CAD build for the part. Positions are in the model's coordinates, mm. A direction names the side the tool comes from. Round coordinates to 2 decimals unless told otherwise and drop trailing zeros. Write each loop counter-clockwise with the first axis right and the second up, starting at its lowest first coordinate (ties: lowest second). Pieces come first, ordered by that corner, then holes. Notation, with made-up numbers: (81.25, 71.25) -> (101.25, 71.25) arc R26 ccw to (101.25, 91.25) -> close; hole circle Ø7 at (14.25, 75.25). An arc over 180 degrees is marked (long way). Put each result on its own line as item: value. Start each with the question number.
1. Saw through at D-D on z = -29. List the corners of the cut face in (x, y) (3 decimals), and give its area (3 significant figures).
2. Pull direction Y, two halves, no side cores. Call faces 1 (the cylindrical face through (-2.21, 39.84, 41.27)), 2 (the flat face through (19.685, 55, 1)), 3 (the flat face through (43, 7.79, -62)): pulls with the +Y half, pulls with the -Y half, needs draft (parallel to the pull), parting line crosses it, or undercut.
3. Flat gauge pins, fed straight in: P1, Ø2.5, axis at x = 2, z = 0.5, coming from the +Y side; P2, Ø8, axis at y = 25.5, z = -16.5, coming from the -X side; P3, Ø9, axis at x = 41.06, z = 60.58, coming from the +Y side. Where does each tip first touch, or does it go through?
4. Saw through at A-A on z = 0. List the corners of the cut face in (x, y) (3 decimals), and give its area (3 significant figures).
5. 3-axis set-ups, long thin cutter, end or side, ignore diameter. For faces 4 (the cylindrical face through (-38.927, 8.88, -63.923)), 5 (the flat face through (0, 61, 43.735)), 6 (the cylindrical face through (28.294, 13.422, -0.78)): which of +Z, -Z, +X, -X, +Y, -Y reach the whole face in a straight line?
6. Saw through at B-B on y = 61.5. List the corners of the cut face in (x, z) (3 decimals).
7. Saw through at C-C on x = 11. List the corners of the cut face in (y, z) (3 decimals).
8. Drill centre lines: line 1 (Y direction, x = 0, z = 41); line 2 (X direction, y = 77, z = -25) (3 decimals); line 3 (Z direction, x = -11.5, y = 26.5) (3 decimals). Where is each one in solid material? Low to high. Write a range as from..to.
from build123d import *

# Parameters (mm, degrees)
SKETCH1_W                                     = 49.37
SKETCH1_H                                     = 87.47
SKETCH1_W_2                                   = 39.37
SKETCH1_H_2                                   = 77.47
BOSS_EXTRUDE1_DEPTH                           = 101.6
SKETCH2_W                                     = 100.17
SKETCH2_H                                     = 138.27
BOSS_EXTRUDE2_DEPTH                           = 10
FILLET1_R                                     = 12
CBORE_FOR_6_BINDING_HEAD_MACHINE_SC_2_R       = 1.89865
CBORE_FOR_6_BINDING_HEAD_MACHINE_SCREW2_DEPTH = 10
CBORE_START                                   = 7.7902
CBORE_FOR_6_BINDING_HEAD_MACHINE_SC_3_O_R     = 3.96875
CBORE_FOR_6_BINDING_HEAD_MACHINE_SC_3_O_R_2   = 1.89865
CBORE_FOR_6_BINDING_HEAD_MACHINE_SC_3_DEPTH   = 2.2098
FILLET2_R                                     = 12
SKETCH9_R                                     = 3
CUT_EXTRUDE1_DEPTH                            = 160.908424184


# Read off the part's stored shape, not the designer's step: CBORE for #6 Binding Head Machine Screw2
with BuildPart() as part:
    # Sketch1 → Boss-Extrude1 (new body)
    with BuildSketch(Plane(origin=(0, 0, 0), x_dir=(1, 0, 0), z_dir=(0, 1, 0))):
        Rectangle(SKETCH1_W, SKETCH1_H)
        Rectangle(SKETCH1_W_2, SKETCH1_H_2, mode=Mode.SUBTRACT)
    extrude(amount=BOSS_EXTRUDE1_DEPTH)

    # Sketch2 → Boss-Extrude2 (add)
    with BuildSketch(Plane(origin=(0, 0, 0), x_dir=(1, 0, 0), z_dir=(0, 1, 0))):
        Rectangle(SKETCH2_W, SKETCH2_H)
    extrude(amount=BOSS_EXTRUDE2_DEPTH)

    # Fillet1
    fillet1_edges = [part.edges().sort_by_distance(p)[0] for p in [
        (0, 10, -43.735),
        (24.685, 10, 0),
        (0, 10, 43.735),
        (-24.685, 10, 0),
    ]]
    fillet(fillet1_edges, radius=FILLET1_R)

    # CBORE for _6 Binding Head Machine Sc 2 → CBORE for #6 Binding Head Machine Screw2 (cut)
    with BuildSketch(Plane(origin=(0, 0, 0), x_dir=(1, 0, 0), z_dir=(0, 1, 0))):
        with Locations((41.060456563, -60.576250035)):
            Circle(CBORE_FOR_6_BINDING_HEAD_MACHINE_SC_2_R)
        with Locations((-41.060456563, 60.576250035)):
            Circle(CBORE_FOR_6_BINDING_HEAD_MACHINE_SC_2_R)
        with Locations((-41.060456563, -60.576250035)):
            Circle(CBORE_FOR_6_BINDING_HEAD_MACHINE_SC_2_R)
        with Locations((41.060456563, 60.576250035)):
            Circle(CBORE_FOR_6_BINDING_HEAD_MACHINE_SC_2_R)
        Circle(CBORE_FOR_6_BINDING_HEAD_MACHINE_SC_2_R)
    extrude(amount=CBORE_FOR_6_BINDING_HEAD_MACHINE_SCREW2_DEPTH, mode=Mode.SUBTRACT)

    # CBORE for _6 Binding Head Machine Sc 3 o → CBORE for _6 Binding Head Machine Sc 3 (cut)
    # profile 1 of 5: a face of its own
    with BuildSketch(Plane(origin=(0, 0, 0), x_dir=(1, 0, 0), z_dir=(0, 1, 0)).offset(CBORE_START)):
        with Locations((41.060456563, -60.576250035)):
            Circle(CBORE_FOR_6_BINDING_HEAD_MACHINE_SC_3_O_R)
        with Locations((41.060456563, -60.576250035)):
            Circle(CBORE_FOR_6_BINDING_HEAD_MACHINE_SC_3_O_R_2, mode=Mode.SUBTRACT)
    # profile 2 of 5: a face of its own
    with BuildSketch(Plane(origin=(0, 0, 0), x_dir=(1, 0, 0), z_dir=(0, 1, 0)).offset(CBORE_START)):
        with Locations((-41.060456563, 60.576250035)):
            Circle(CBORE_FOR_6_BINDING_HEAD_MACHINE_SC_3_O_R)
        with Locations((-41.060456563, 60.576250035)):
            Circle(CBORE_FOR_6_BINDING_HEAD_MACHINE_SC_3_O_R_2, mode=Mode.SUBTRACT)
    # profile 3 of 5: a face of its own
    with BuildSketch(Plane(origin=(0, 0, 0), x_dir=(1, 0, 0), z_dir=(0, 1, 0)).offset(CBORE_START)):
        with Locations((-41.060456563, -60.576250035)):
            Circle(CBORE_FOR_6_BINDING_HEAD_MACHINE_SC_3_O_R)
        with Locations((-41.060456563, -60.576250035)):
            Circle(CBORE_FOR_6_BINDING_HEAD_MACHINE_SC_3_O_R_2, mode=Mode.SUBTRACT)
    # profile 4 of 5: a face of its own
    with BuildSketch(Plane(origin=(0, 0, 0), x_dir=(1, 0, 0), z_dir=(0, 1, 0)).offset(CBORE_START)):
        with Locations((41.060456563, 60.576250035)):
            Circle(CBORE_FOR_6_BINDING_HEAD_MACHINE_SC_3_O_R)
        with Locations((41.060456563, 60.576250035)):
            Circle(CBORE_FOR_6_BINDING_HEAD_MACHINE_SC_3_O_R_2, mode=Mode.SUBTRACT)
    # profile 5 of 5: a face of its own
    with BuildSketch(Plane(origin=(0, 0, 0), x_dir=(1, 0, 0), z_dir=(0, 1, 0)).offset(CBORE_START)):
        Circle(CBORE_FOR_6_BINDING_HEAD_MACHINE_SC_3_O_R)
        Circle(CBORE_FOR_6_BINDING_HEAD_MACHINE_SC_3_O_R_2, mode=Mode.SUBTRACT)
    extrude(amount=CBORE_FOR_6_BINDING_HEAD_MACHINE_SC_3_DEPTH, mode=Mode.SUBTRACT)

    # Fillet2
    fillet2_edges = [part.edges().sort_by_distance(p)[0] for p in [
        (50.085, 5, 69.135),
        (50.085, 5, -69.135),
        (-50.085, 5, -69.135),
        (-50.085, 5, 69.135),
    ]]
    fillet(fillet2_edges, radius=FILLET2_R)

    # Sketch9 → Cut-Extrude1 (cut, through all)
    with BuildSketch(Plane.XY.offset(43.735)):
        with Locations((0, 88.608727906)):
            Circle(SKETCH9_R)
        with Locations((0, 37.808727906)):
            Circle(SKETCH9_R)
    extrude(amount=-CUT_EXTRUDE1_DEPTH, mode=Mode.SUBTRACT)


solid = part.part
Return value:
1. outline: (-50.085, 0) -> (50.085, 0) -> (50.085, 10) -> (36.685, 10) arc R12 cw to (24.685, 22) -> (24.685, 101.6) -> (19.685, 101.6) -> (19.685, 10) -> (-19.685, 10) -> (-19.685, 101.6) -> (-24.685, 101.6) -> (-24.685, 22) arc R12 cw to (-36.685, 10) -> (-50.085, 10) -> close
1. area: 1,980 mm^2
2. face 1: undercut
2. face 2: needs draft
2. face 3: pulls with the +Y half
3. P1: stops at y = 7.79
3. P2: stops at x = -24.7
3. P3: stops at y = 10
4. outline: (-50.085, 0) -> (-1.899, 0) -> (-1.899, 7.79) -> (-3.969, 7.79) -> (-3.969, 10) -> (-19.685, 10) -> (-19.685, 101.6) -> (-24.685, 101.6) -> (-24.685, 22) arc R12 cw to (-36.685, 10) -> (-50.085, 10) -> close; (1.899, 0) -> (50.085, 0) -> (50.085, 10) -> (36.685, 10) arc R12 cw to (24.685, 22) -> (24.685, 101.6) -> (19.685, 101.6) -> (19.685, 10) -> (3.969, 10) -> (3.969, 7.79) -> (1.899, 7.79) -> close
4. area: 1,930 mm^2
5. face 4: +Y
5. face 5: +Z, +X, -X, +Y
5. face 6: +Z, -Z, +X, +Y
6. outline: (-24.685, -43.735) -> (24.685, -43.735) -> (24.685, 43.735) -> (-24.685, 43.735) -> close; hole (-19.685, -38.735) -> (19.685, -38.735) -> (19.685, 38.735) -> (-19.685, 38.735) -> close
7. outline: (0, -69.135) -> (10, -69.135) -> (10, -55.735) arc R12 cw to (22, -43.735) -> (101.6, -43.735) -> (101.6, -38.735) -> (10, -38.735) -> (10, 38.735) -> (101.6, 38.735) -> (101.6, 43.735) -> (22, 43.735) arc R12 cw to (10, 55.735) -> (10, 69.135) -> (0, 69.135) -> close
8. line 1: y = 0..34.81, 40.81..85.61, 91.61..101.6
8. line 2: x = -24.685..-19.685, 19.685..24.685
8. line 3: z = -43.735..-38.735, 38.735..43.735
